Source: CAD feature listing. Evaluate the final solid. Frame: model axes, mm. A direction names the side the tool comes from. Give positions to 0.01 mm unless a question says otherwise; leave off trailing zeros. Loops run counter-clockwise (first coordinate to the right, second up) from the corner with the lowest first, then second, coordinate; pieces in that order, holes last. Notation, with made-up numbers: (37.5, 50.5) -> (88.5, 50.5) arc R37 ccw to (88.5, 86.5) -> close; hole circle Ø3 at (65, 32). An arc over 180 degrees is marked (long way). Answer as a JSON object with one key per item and string values. Group by question number.
from build123d import *

# Parameters (mm, degrees)
F0_W     = 50
F0_H     = 50
F1_DEPTH = 50
F2_R     = 15
F3_SIZE  = 5
F4_T     = -2.5


with BuildPart() as f1:
    # F0 (on Top) → F1 (new body)
    with BuildSketch(Plane.XY):
        Rectangle(F0_W, F0_H)
    extrude(amount=F1_DEPTH)

    # F2
    f2_edges = [f1.edges().sort_by_distance(p)[0] for p in [
        (-25, -25, 25),
        (25, -25, 25),
        (25, 25, 25),
        (-25, 25, 25),
    ]]
    fillet(f2_edges, radius=F2_R)

    # F3
    f3_edges = [f1.edges().sort_by_distance(p)[0] for p in [
        (20.606602, 20.606602, 0),
        (20.606602, -20.606602, 0),
        (-20.606602, -20.606602, 0),
        (-20.606602, 20.606602, 0),
    ]]
    chamfer(f3_edges, length=F3_SIZE)

    # F4
    f4_openings = [f1.faces().sort_by_distance(p)[0] for p in [
        (0, 0, 50),
    ]]
    offset(amount=F4_T, openings=f4_openings)


solid = f1.part
(1) Material intervals for line 1 (X direction, y = 0, z = 13); line 2 (Y direction, x = -14, z = 8), sorted ascending. Write a range as from..to.
(2) Access query for faces 1 (the face through (18.38, -18.56, 1.98)), 2 (the face through (18.935, 18.741, 28.326)). Directions: +Z, -Z, +X, -X, +Y, -Y. A direction counts if a zero-diameter tool reaches every point of the face in a straight line with its end or side. Return the directions, or none.
(3) Section query B-B on y = -7.5. Return the cut outline in (x, z).
(4) First-contact query: pin 1 (4 mm diameter, centred on x = 18.5, y = 15.5, fed in from -Z); pin 2 (8 mm diameter, centred on y = 19.5, z = 42.5, fed in from -X); pin 3 (3 mm diameter, centred on x = -10.5, y = 20, fed in from +Z); pin 4 (10 mm diameter, centred on x = 4.5, y = 12.5, fed in from +Z). Flat tips, straight axial feed; report the tip coordinate or a pass-through.
(5) Section query A-A on z = 46.5. Return the cut outline in (x, y), plus the area to 3 significant figures.
(6) Mould query, pull axis Y, two halves, no side actions, for faces 3 (the face through (-20.757, 0.14, 4.293)), 4 (the face through (-18.56, -18.38, 1.98)), 5 (the face through (25, 0, 27)). Classes: pulls with the +Y half, pulls with the -Y half, needs draft (parallel to the pull), parting line crosses it, or undercut.
Result:
{
 "1": {"line 1": "-25..-22.5, 22.5..25", "line 2": "-24.46..-21.84, 21.84..24.46"},
 "2": {"face 1": "-Z, +X, -Y", "face 2": "+Z"},
 "3": {"outline": "(-25, 5) -> (-20, 0) -> (20, 0) -> (25, 5) -> (25, 50) -> (22.5, 50) -> (22.5, 6.04) -> (18.96, 2.5) -> (-18.96, 2.5) -> (-22.5, 6.04) -> (-22.5, 50) -> (-25, 50) -> close"},
 "4": {"pin 1": "z = 0", "pin 2": "x = -23.96", "pin 3": "z = 5.05", "pin 4": "z = 2.5"},
 "5": {"outline": "(-25, -10) arc R15 ccw to (-10, -25) -> (10, -25) arc R15 ccw to (25, -10) -> (25, 10) arc R15 ccw to (10, 25) -> (-10, 25) arc R15 ccw to (-25, 10) -> close; hole (-22.5, -10) arc R12.5 ccw to (-10, -22.5) -> (10, -22.5) arc R12.5 ccw to (22.5, -10) -> (22.5, 10) arc R12.5 ccw to (10, 22.5) -> (-10, 22.5) arc R12.5 ccw to (-22.5, 10) -> close", "area": "416 mm²"},
 "6": {"face 3": "undercut", "face 4": "pulls with the -Y half", "face 5": "needs draft"}
}
